Model file for the job. Use its own axes, mm. A direction names the side the tool comes from. Coordinates: 2 decimals unless noted, no trailing zeros. Order: outer loops, then holes, each group sorted by start corner. A loop starts at its lowest first (then second) coordinate and runs counter-clockwise, first axis right, second up.
from build123d import *

# Parameters (mm, degrees)
SKETCH2_W           = 55
SKETCH2_H           = 80
BOSS_EXTRUDE1_DEPTH = 50
SKETCH4_R           = 4
CUT_EXTRUDE1_DEPTH  = 110.201648339
SKETCH5_R           = 4.075
CUT_EXTRUDE2_DEPTH  = 8.03
SKETCH6_W           = 35
SKETCH6_H           = 21
CUT_EXTRUDE3_DEPTH  = 32
SKETCH10_R          = 6.75
CUT_EXTRUDE5_DEPTH  = 26.55
CUT_EXTRUDE6_DEPTH  = 26.55
SKETCH12_R          = 2
CUT_EXTRUDE7_DEPTH  = 5
SKETCH13_R          = 2.1
CUT_EXTRUDE8_DEPTH  = 103.220350224
SKETCH13_3_R        = 3.75
CUT_EXTRUDE9_DEPTH  = 4.5
SKETCH14_R          = 2.25
CUT_EXTRUDE10_DEPTH = 10
SKETCH15_W          = 4
SKETCH15_H          = 8
CUT_EXTRUDE11_DEPTH = 13
CUT_EXTRUDE12_DEPTH = 0.5


with BuildPart() as part:
    # Sketch2 → Boss-Extrude1 (new body)
    with BuildSketch(Plane.XY):
        with Locations((27.5, 40)):
            Rectangle(SKETCH2_W, SKETCH2_H)
    extrude(amount=BOSS_EXTRUDE1_DEPTH)

    # Sketch4 → Cut-Extrude1 (cut, through all)
    with BuildSketch(Plane(origin=(0, 80, 0), x_dir=(1, 0, 0), z_dir=(0, 1, 0))):
        with Locations(Location((40, -34, 0), (0, 0, 270))):
            Circle(SKETCH4_R)
    extrude(amount=-CUT_EXTRUDE1_DEPTH, mode=Mode.SUBTRACT)

    # Sketch5 → Cut-Extrude2 (cut)
    with BuildSketch(Plane.XY.offset(50)):
        with Locations((21, 71)):
            Circle(SKETCH5_R)
        with Locations((21, 9)):
            Circle(SKETCH5_R)
    extrude(amount=-CUT_EXTRUDE2_DEPTH, mode=Mode.SUBTRACT)

    # Sketch6 → Cut-Extrude3 (cut)
    with BuildSketch(Plane.XY.offset(50)):
        with Locations((37.5, 40)):
            Rectangle(SKETCH6_W, SKETCH6_H)
    extrude(amount=-CUT_EXTRUDE3_DEPTH, mode=Mode.SUBTRACT)

    # Sketch10 → Cut-Extrude5 (cut)
    with BuildSketch(Plane(origin=(0, 80, 0), x_dir=(1, 0, 0), z_dir=(0, 1, 0))):
        with Locations(Location((40, -34, 0), (0, 0, 270))):
            Circle(SKETCH10_R)
    extrude(amount=-CUT_EXTRUDE5_DEPTH, mode=Mode.SUBTRACT)

    # Sketch11 → Cut-Extrude6 (cut)
    with BuildSketch(Plane.XZ):
        Polygon((47.563288526, 34), (43.781644263, 40.55), (36.218355737, 40.55), (32.436711474, 34), (36.218355737, 27.45), (43.781644263, 27.45), align=None)
    extrude(amount=-CUT_EXTRUDE6_DEPTH, mode=Mode.SUBTRACT)

    # Sketch12 → Cut-Extrude7 (cut)
    with BuildSketch(Plane.XZ):
        with Locations(Location((12.5, 7.5, 0), (0, 0, 270))):
            Circle(SKETCH12_R)
        with Locations(Location((12.5, 22.5, 0), (0, 0, 270))):
            Circle(SKETCH12_R)
    extrude(amount=-CUT_EXTRUDE7_DEPTH, mode=Mode.SUBTRACT)

    # Sketch13 → Cut-Extrude8 (cut, through all)
    with BuildSketch(Plane.XY.offset(18)):
        with Locations((27.5, 40)):
            Circle(SKETCH13_R)
        with Locations((47.5, 40)):
            Circle(SKETCH13_R)
    extrude(amount=-CUT_EXTRUDE8_DEPTH, mode=Mode.SUBTRACT)

    # Sketch13<3> → Cut-Extrude9 (cut)
    with BuildSketch(Plane.XY.offset(18)):
        with Locations((27.5, 40)):
            Circle(SKETCH13_3_R)
        with Locations((47.5, 40)):
            Circle(SKETCH13_3_R)
    extrude(amount=-CUT_EXTRUDE9_DEPTH, mode=Mode.SUBTRACT)

    # Sketch14 → Cut-Extrude10 (cut)
    with BuildSketch(Plane.ZY):
        with Locations((30, 72)):
            Circle(SKETCH14_R)
    extrude(amount=-CUT_EXTRUDE10_DEPTH, mode=Mode.SUBTRACT)

    # Sketch15 → Cut-Extrude11 (cut)
    with BuildSketch(Plane(origin=(0, 80, 0), x_dir=(1, 0, 0), z_dir=(0, 1, 0))):
        with Locations((7, -30)):
            Rectangle(SKETCH15_W, SKETCH15_H)
    extrude(amount=-CUT_EXTRUDE11_DEPTH, mode=Mode.SUBTRACT)

    # Sketch16 → Cut-Extrude12 (cut)
    with BuildSketch(Plane(origin=(55, 0, 0), x_dir=(0, 0, -1), z_dir=(1, 0, 0))):
        with BuildLine():
            Line((-27.692307692, 75.25), (-25.741185897, 75.25))
            add(Edge.make_bspline(
                [(-25.741185897, 75.25), (-25.64567596, 75.249497856), (-25.46055393, 75.248524576), (-25.191355525, 75.233429916), (-24.939216066, 75.212848002), (-24.704062431, 75.180190594), (-24.486003281, 75.140785516), (-24.28438146, 75.093066042), (-24.099838111, 75.035847146), (-23.879516007, 74.944857771), (-23.628314119, 74.809648718), (-23.356318711, 74.609852818), (-23.12373517, 74.365474352), (-22.923202835, 74.089809622), (-22.763771065, 73.78656456), (-22.648430215, 73.462966878), (-22.575407714, 73.123190472), (-22.567897902, 72.88992425), (-22.564102564, 72.772035256)],
                knots=[0, 0, 0, 0, 1.001505555, 1.941167018, 2.826882275, 3.653841531, 4.429895133, 5.150066043, 5.825578002, 6.45369114, 7.647487171, 8.808567382, 9.977351308, 11.170798116, 12.373658725, 13.556498008, 14.765093433, 16, 16, 16, 16], degree=3))
            add(Edge.make_bspline(
                [(-22.564102564, 72.772035256), (-22.567226045, 72.661599383), (-22.573363981, 72.444582477), (-22.632057579, 72.127170736), (-22.723945203, 71.825024397), (-22.851674486, 71.539246153), (-23.01768019, 71.276292972), (-23.214418243, 71.034043641), (-23.451780536, 70.822754907), (-23.629618364, 70.704632328), (-23.719951923, 70.64463141)],
                knots=[0, 0, 0, 0, 1.044552857, 2.05264487, 3.044412934, 4.028983338, 5.005914585, 5.980388656, 6.974128949, 8, 8, 8, 8], degree=3))
            add(Edge.make_bspline(
                [(-23.719951923, 70.64463141), (-23.606350701, 70.601017128), (-23.389003423, 70.517572201), (-23.08990053, 70.370042304), (-22.832200973, 70.209579131), (-22.613923413, 70.034345273), (-22.427244399, 69.845462957), (-22.264235995, 69.640162631), (-22.125146354, 69.415766179), (-22.005966573, 69.174613221), (-21.912970127, 68.919166169), (-21.843324686, 68.651821094), (-21.803417688, 68.373536651), (-21.797738713, 68.184149853), (-21.794871795, 68.088541667)],
                knots=[0, 0, 0, 0, 1.27268992, 2.434971085, 3.483601985, 4.442670788, 5.356604649, 6.2567628, 7.179492994, 8.113709626, 9.066344395, 10.018646069, 10.999752585, 12, 12, 12, 12], degree=3))
            add(Edge.make_bspline(
                [(-21.794871795, 68.088541667), (-21.797662784, 67.990922032), (-21.803154132, 67.798852666), (-21.843668337, 67.516695139), (-21.912265786, 67.247052434), (-22.006754775, 66.988180484), (-22.130075674, 66.740580099), (-22.280155572, 66.503970774), (-22.459102897, 66.280729829), (-22.659282522, 66.06837662), (-22.885745795, 65.877440085), (-23.130076523, 65.707395209), (-23.395351723, 65.567549317), (-23.677214563, 65.45007497), (-23.978826895, 65.360340117), (-24.298834345, 65.297561334), (-24.636960921, 65.255261229), (-24.868988782, 65.2517835), (-24.987980769, 65.25)],
                knots=[0, 0, 0, 0, 0.978564426, 1.925352924, 2.850884081, 3.763762016, 4.682927383, 5.618979971, 6.567305752, 7.547517671, 8.540179244, 9.531824382, 10.526200242, 11.540722885, 12.589160233, 13.674978461, 14.80764778, 16, 16, 16, 16], degree=3))
            Line((-24.987980769, 65.25), (-27.692307692, 65.25))
            Line((-27.692307692, 65.25), (-27.692307692, 75.25))
        make_face()
        with BuildLine():
            Line((-26.794871795, 74.224358974), (-26.794871795, 71.019230769))
            Line((-26.794871795, 71.019230769), (-26.191907051, 71.019230769))
            add(Edge.make_bspline(
                [(-26.191907051, 71.019230769), (-26.103767636, 71.020373406), (-25.933464324, 71.022581214), (-25.686836048, 71.028905549), (-25.457907424, 71.046614244), (-25.247073616, 71.06431785), (-25.054666633, 71.093102386), (-24.881112743, 71.127365595), (-24.72368818, 71.163602466), (-24.542146622, 71.225229572), (-24.336223912, 71.316308644), (-24.116700757, 71.457656747), (-23.923173701, 71.626012042), (-23.759753165, 71.820271932), (-23.626006106, 72.034175321), (-23.533109777, 72.264309265), (-23.470117536, 72.504938213), (-23.464427447, 72.670133221), (-23.461538462, 72.75400641)],
                knots=[0, 0, 0, 0, 1.156816544, 2.235205308, 3.236616184, 4.169592532, 5.011045266, 5.787822928, 6.49130361, 7.128639758, 8.301311294, 9.436451833, 10.541879658, 11.654887649, 12.756523258, 13.837046038, 14.901820046, 16, 16, 16, 16], degree=3))
            add(Edge.make_bspline(
                [(-23.461538462, 72.75400641), (-23.463041833, 72.809508615), (-23.465990862, 72.918382249), (-23.490143155, 73.07709469), (-23.531193368, 73.226362554), (-23.58391992, 73.368231441), (-23.657601887, 73.498265298), (-23.74435464, 73.620960143), (-23.849170898, 73.732137625), (-23.968477505, 73.836050477), (-24.105644999, 73.928177699), (-24.260591547, 74.008865594), (-24.435413482, 74.073839242), (-24.627164496, 74.130742534), (-24.838796175, 74.170709088), (-25.067866327, 74.204004482), (-25.316251239, 74.220955173), (-25.488094389, 74.223199067), (-25.576923077, 74.224358974)],
                knots=[0, 0, 0, 0, 0.91205012, 1.789085906, 2.630437955, 3.453916878, 4.269457761, 5.079663411, 5.91843418, 6.774407191, 7.675494373, 8.627863946, 9.638891023, 10.736472738, 11.911756761, 13.175263542, 14.539845004, 16, 16, 16, 16], degree=3))
            Line((-25.576923077, 74.224358974), (-26.794871795, 74.224358974))
        make_face(mode=Mode.SUBTRACT)
        with BuildLine():
            Line((-26.794871795, 69.993589744), (-26.794871795, 66.275641026))
            Line((-26.794871795, 66.275641026), (-25.516826923, 66.275641026))
            add(Edge.make_bspline(
                [(-25.516826923, 66.275641026), (-25.425344278, 66.276737447), (-25.249023539, 66.278850654), (-24.994448596, 66.285749381), (-24.75849687, 66.301441598), (-24.542245054, 66.326144025), (-24.343358047, 66.352939594), (-24.164221752, 66.388971825), (-24.003384057, 66.43025457), (-23.816886034, 66.49406649), (-23.606876011, 66.593199265), (-23.380559278, 66.742668483), (-23.179341512, 66.920735076), (-23.008469343, 67.126823403), (-22.868432233, 67.350912908), (-22.766559504, 67.588471051), (-22.703728485, 67.835572558), (-22.696122287, 68.004048879), (-22.692307692, 68.088541667)],
                knots=[0, 0, 0, 0, 1.160039823, 2.235823828, 3.228722157, 4.157150951, 4.99529583, 5.772374946, 6.472645482, 7.099169577, 8.269452708, 9.405989375, 10.527446681, 11.663510218, 12.788923519, 13.866172445, 14.929861265, 16, 16, 16, 16], degree=3))
            add(Edge.make_bspline(
                [(-22.692307692, 68.088541667), (-22.693096562, 68.141379782), (-22.694661576, 68.24620373), (-22.718263333, 68.400248928), (-22.752588676, 68.549465709), (-22.796964201, 68.694259253), (-22.86159125, 68.832011757), (-22.937038521, 68.965447641), (-23.025499669, 69.094743297), (-23.163340143, 69.258206878), (-23.363831527, 69.446541201), (-23.648708028, 69.630934064), (-23.97262888, 69.779642085), (-24.207564574, 69.842783446), (-24.328926282, 69.875400641)],
                knots=[0, 0, 0, 0, 0.723448775, 1.435228256, 2.130040452, 2.821711965, 3.505591119, 4.210454504, 4.921174351, 5.648778258, 7.137944449, 8.670945889, 10.280296675, 12, 12, 12, 12], degree=3))
            add(Edge.make_bspline(
                [(-24.328926282, 69.875400641), (-24.377580842, 69.885272309), (-24.483073963, 69.906676123), (-24.655095621, 69.929269561), (-24.851483818, 69.949398304), (-25.072692039, 69.964287326), (-25.319000156, 69.97967745), (-25.590934209, 69.985662653), (-25.88738368, 69.992803396), (-26.093076172, 69.993320923), (-26.199919872, 69.993589744)],
                knots=[0, 0, 0, 0, 0.634451884, 1.375622551, 2.216452059, 3.157844607, 4.20941857, 5.370758133, 6.634282058, 8, 8, 8, 8], degree=3))
            Line((-26.199919872, 69.993589744), (-26.794871795, 69.993589744))
        make_face(mode=Mode.SUBTRACT)
    extrude(amount=-CUT_EXTRUDE12_DEPTH, mode=Mode.SUBTRACT)


solid = part.part
Q1. Cut at C-C, the plane z = 17. List the corners of the cut face in (x, y).
Established:
outline: (0, 0) - (55, 0) - (55, 80) - (0, 80) - close; hole circle Ø7.5 at (27.5, 40); hole circle Ø7.5 at (47.5, 40)
Q2. Cut at A-A, the plane y = 18.5. List the corners of the cut face in (x, z), plus the area to 3 significant figures.
Established:
outline: (0, 0) - (55, 0) - (55, 50) - (0, 50) - close; hole (32.44, 34) - (36.22, 27.45) - (43.78, 27.45) - (47.56, 34) - (43.78, 40.55) - (36.22, 40.55) - close
area: 2,600 mm2
Q3. Mould opens along X. For faces 5 (the face through (9, 75, 30)), 6 (the face through (9.493, 69.804, 29.512)), 7 (the face through (22.88, 5.385, 46.041)), 8 (the face through (20, 40, 34)) say: pulls with the +X half, pulls with the -X half, needs draft (parallel to the pull), parting line crosses it, or undercut.
Established:
face 5: undercut
face 6: needs draft
face 7: undercut
face 8: pulls with the +X half
Q4. Probe line 1 (Y direction, x = 9.7, z = 30); line 2 (X direction, y = 51.2, z = 34); line 3 (Y direction, x = 25.5, z = 19). List the from-to ranges inside material, lowest first.
Established:
line 1: y = 0 to 69.75, 74.25 to 80
line 2: x = 0 to 36, 44 to 55
line 3: y = 0 to 29.5, 50.5 to 80
Q5. Drop flat-ended pins along their axis: P1, Ø13, axis at x = 40, z = 34, coming from the +Y side; P2, Ø3, axis at y = 38.5, z = 44, coming from the +X side; P3, Ø3.5, axis at y = 72, z = 30, coming from the -X side; P4, Ø2, axis at x = 28.5, y = 40, coming from the +Z side. Give the stop position or say it passes through.
Established:
P1: stops at y = 53.45
P2: stops at x = 20
P3: stops at x = 10
P4: passes through
Q6. Cut at B-B, the plane x = 40. List the corners of the cut face in (y, z), plus the area to 3 significant figures.
Established:
outline: (0, 0) - (80, 0) - (80, 27.25) - (53.45, 27.25) - (53.45, 30) - (50.5, 30) - (50.5, 18) - (29.5, 18) - (29.5, 30) - (26.55, 30) - (26.55, 27.45) - (0, 27.45) - close; (0, 40.55) - (26.55, 40.55) - (26.55, 38) - (29.5, 38) - (29.5, 50) - (0, 50) - close; (50.5, 38) - (53.45, 38) - (53.45, 40.75) - (80, 40.75) - (80, 50) - (50.5, 50) - close
area: 2,570 mm2
Q7. Which spindle directions (+Z, -Z, +X, -X, +Y, -Y) get a long thin tool onto all of the face, cutting with end or side? Do faces 1 (the face through (21, 71, 41.97)), 2 (the face through (45.7, 13.09, 37.23)), 3 (the face through (37, 53.45, 37)), 4 (the face through (15, 41, 50)). Say none if no direction does.
Established:
face 1: +Z
face 2: -Y
face 3: +Y
face 4: +Z, +X, -X, +Y, -Y
Q8. Cut at D-D, the plane y = 9. List the corners of the cut face in (x, z) (3 decimals).
Established:
outline: (0, 0) - (55, 0) - (55, 50) - (25.075, 50) - (25.075, 41.97) - (16.925, 41.97) - (16.925, 50) - (0, 50) - close; hole (32.437, 34) - (36.218, 27.45) - (43.782, 27.45) - (47.563, 34) - (43.782, 40.55) - (36.218, 40.55) - close
